For this review, take the finished solid that the model builds, in its own axes (mm). A direction names the side the tool comes from. Give positions to 0.01 mm unless a question says otherwise; leave off trailing zeros. Loops run counter-clockwise (first coordinate to the right, second up) from the corner with the lowest first, then second, coordinate; pieces in that order, holes last. Notation, with made-up numbers: (89, 64.25) - (97, 64.25) arc R19 cw to (97, 90.25) - close; hole circle Ø10 at (-37, 80). An arc over 180 degrees is marked (long way). Answer in a Markdown table with one row per item.
```python
from build123d import *

# Parameters (mm, degrees)
F0_R             = 11
F1_DEPTH         = 1.905
F3_R             = 2.54
F4_DEPTH         = 3.175
F4_COPIES2_COUNT = 2
F5_R             = 2.54


# Not quite as in the source:
# - a pattern or mirror of a feature is missing from the dataset's text; its kind, count and spacing are read off the source's solid


with BuildPart() as f1:
    # F0 (on Top) → F1 (new body, symmetric)
    with BuildSketch(Plane.XY):
        with BuildLine():
            Line((-31.75, -6.9869237544), (-2.3327823548, -12.4839147099))
            ThreePointArc((-2.3327823548, -12.4839147099), (0, -12.7), (2.3327823548, -12.4839147099))
            Line((2.3327823548, -12.4839147099), (31.75, -6.9869237544))
            Line((31.75, -6.9869237544), (31.75, 6.9869237544))
            Line((31.75, 6.9869237544), (2.3327823548, 12.4839147099))
            ThreePointArc((2.3327823548, 12.4839147099), (0, 12.7), (-2.3327823548, 12.4839147099))
            Line((-2.3327823548, 12.4839147099), (-31.75, 6.9869237544))
            Line((-31.75, 6.9869237544), (-31.75, -6.9869237544))
        make_face()
        Circle(F0_R, mode=Mode.SUBTRACT)
    extrude(amount=F1_DEPTH, both=True)

    # F3
    f3_edges = [f1.edges().sort_by_distance(p)[0] for p in [
        (-31.75, 6.986924, 0),
        (-31.75, -6.986924, 0),
        (31.75, -6.986924, 0),
        (31.75, 6.986924, 0),
    ]]
    fillet(f3_edges, radius=F3_R)

    # F2 (on face) → F4 (join)
    with BuildSketch(Plane.XY.offset(1.905)):
        Polygon((-29.21, 4.8775907903), (-29.21, -4.8775907903), (-14.175, -7.6870767183), (-14.175, 7.6870767183), align=None)
    f4 = extrude(amount=F4_DEPTH)

    # F4_copies: F4 across plane
    add(f4.mirror(Plane(origin=(0, 0, 0), x_dir=(0, 0, 1), z_dir=(1, 0, 0))))

    # F4_copies1: F4 across plane
    add(f4.mirror(Plane(origin=(0, 0, 0), x_dir=(-1, 0, 0), z_dir=(0, 0, -1))))

    # F4_copies2: F4 ×2 about axis
    f4_copies2_axis = Axis((0, 0, 0), (0, 1, 0))
    for i in range(1, F4_COPIES2_COUNT):
        add(f4.rotate(f4_copies2_axis, i * 360 / F4_COPIES2_COUNT))

    # F5
    f5_edges = [f1.edges().sort_by_distance(p)[0] for p in [
        (-29.21, -4.877591, 3.4925),
        (-14.175, -7.687077, 3.4925),
        (-14.175, 7.687077, 3.4925),
        (-29.21, 4.877591, 3.4925),
        (-14.175, -7.687077, -3.4925),
        (-14.175, 7.687077, -3.4925),
        (-29.21, -4.877591, -3.4925),
        (-29.21, 4.877591, -3.4925),
        (29.21, -4.877591, -3.4925),
        (14.175, -7.687077, -3.4925),
        (29.21, 4.877591, -3.4925),
        (14.175, 7.687077, -3.4925),
        (29.21, -4.877591, 3.4925),
        (14.175, -7.687077, 3.4925),
        (29.21, 4.877591, 3.4925),
        (14.175, 7.687077, 3.4925),
    ]]
    fillet(f5_edges, radius=F5_R)


solid = f1.part
```
1. Wall thickness on line 1 (Y direction, x = 0, z = 0.4); line 2 (X direction, y = 1, z = 4) (3 decimals); line 3 (X direction, y = -4, z = 1): over which ranges is each line inside the solid? List them lowest first. Write a range as [from, to].
Values:
| item | result |
|---|---|
| line 1 | y = [-12.7, -11], [11, 12.7] |
| line 2 | x = [-29.21, -14.175], [14.175, 29.21] |
| line 3 | x = [-31.75, -10.25], [10.25, 31.75] |
2. We need section D-D, the plane y = 8. Give the boundary of the cut face in (x, z) (1 decimal).
Values:
| item | result |
|---|---|
| outline | (-26.3, -1.9) - (-7.5, -1.9) - (-7.5, 1.9) - (-26.3, 1.9) - close; (7.5, -1.9) - (26.3, -1.9) - (26.3, 1.9) - (7.5, 1.9) - close |
3. We need section B-B, the plane x = 0. Give the boundary of the cut face in (y, z) (3 decimals).
Values:
| item | result |
|---|---|
| outline | (-12.7, -1.905) - (-11, -1.905) - (-11, 1.905) - (-12.7, 1.905) - close; (11, -1.905) - (12.7, -1.905) - (12.7, 1.905) - (11, 1.905) - close |
4. For faces 1 (the face through (-15.116, 6.602, -3.515)), 2 (the face through (-15.116, -6.602, 3.515)), 3 (the face through (14.175, 0, -3)), list the 3-axis set-ups (+Z, -Z, +X, -X, +Y, -Y) from which the entire face can be reached by the end or side of a thin tool; tool diameter is ignored.
Values:
| item | result |
|---|---|
| face 1 | -Z, +Y |
| face 2 | +Z, -Y |
| face 3 | -Z, +Y, -Y |
5. We need section C-C, the plane y = 0. Give the boundary of the cut face in (x, z) (3 decimals).
Values:
| item | result |
|---|---|
| outline | (-31.75, -1.905) - (-29.21, -1.905) - (-29.21, -5.08) - (-14.175, -5.08) - (-14.175, -1.905) - (-11, -1.905) - (-11, 1.905) - (-14.175, 1.905) - (-14.175, 5.08) - (-29.21, 5.08) - (-29.21, 1.905) - (-31.75, 1.905) - close; (11, -1.905) - (14.175, -1.905) - (14.175, -5.08) - (29.21, -5.08) - (29.21, -1.905) - (31.75, -1.905) - (31.75, 1.905) - (29.21, 1.905) - (29.21, 5.08) - (14.175, 5.08) - (14.175, 1.905) - (11, 1.905) - close |
6. We need section A-A, the plane z = -4.25. Give the boundary of the cut face in (x, y) (3 decimals).
Values:
| item | result |
|---|---|
| outline | (-29.21, -2.768) arc R2.54 ccw to (-27.137, -5.265) - (-17.182, -7.125) arc R2.54 ccw to (-14.175, -4.628) - (-14.175, 4.628) arc R2.54 ccw to (-17.182, 7.125) - (-27.137, 5.265) arc R2.54 ccw to (-29.21, 2.768) - close; (14.175, -4.628) arc R2.54 ccw to (17.182, -7.125) - (27.137, -5.265) arc R2.54 ccw to (29.21, -2.768) - (29.21, 2.768) arc R2.54 ccw to (27.137, 5.265) - (17.182, 7.125) arc R2.54 ccw to (14.175, 4.628) - close |
7. Mouldability with a two-part tool opening along X and no side actions: class faces 4 (the face through (28.61, 4.41, -3.51)), 5 (the face through (-14.175, 0, 3)), 6 (the face through (-31.15, -6.52, -0.03)) as released by +X, released by -X, zero draft, split by the parting line, or undercut.
Values:
| item | result |
|---|---|
| face 4 | released by +X |
| face 5 | undercut |
| face 6 | released by -X |
8. Clearance check with flat-ended pins moving along their axes: pin 1 (1 mm diameter, centred on y = 1, z = 3, fed in from +X); pin 2 (1.6 mm diameter, centred on y = 1, z = -4, fed in from -X); pin 3 (5 mm diameter, centred on y = 8, z = -4, fed in from +X). State where each tip first meets the part, or that it passes through.
Values:
| item | result |
|---|---|
| pin 1 | stops at x = 29.21 |
| pin 2 | stops at x = -29.21 |
| pin 3 | stops at x = 31.04 |
